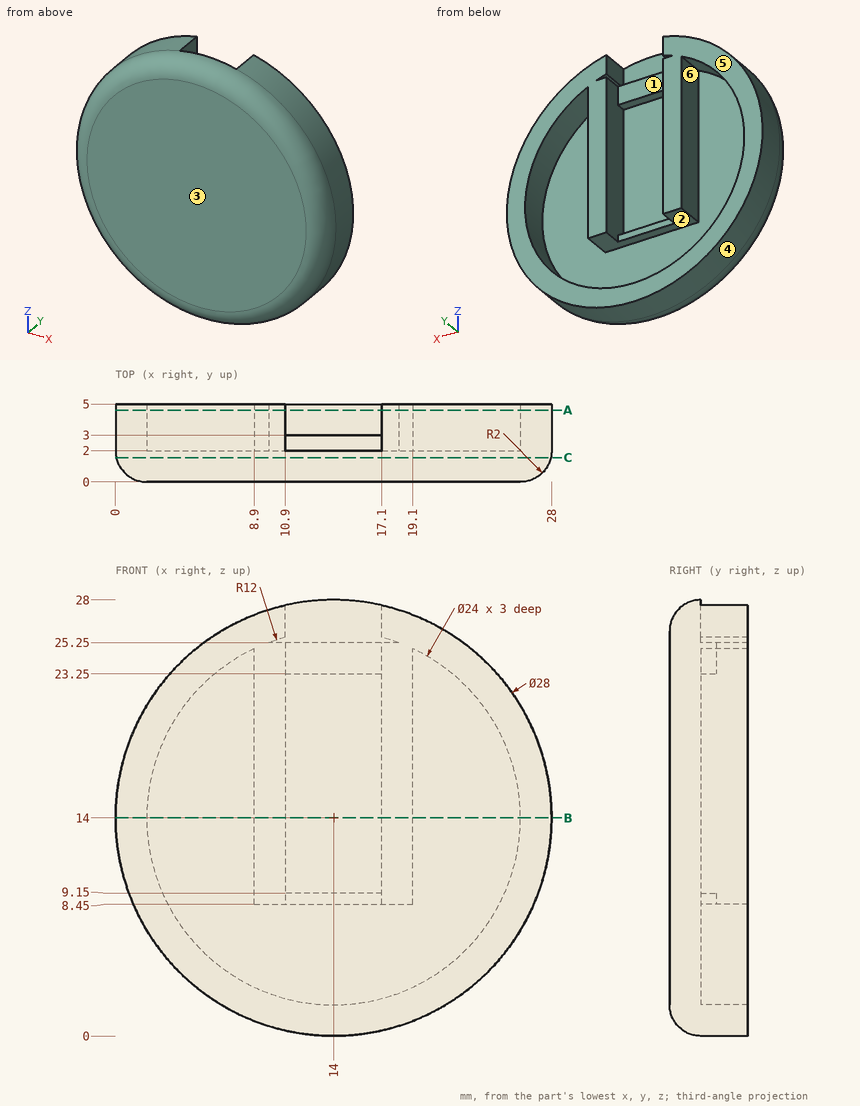
Answer from the drawing. Dimensions are ordinates in mm from the lowest x, y and z of the part. A direction names the side the tool comes from. Give positions to 0.01 mm unless a question says otherwise; leave off trailing zeros. Write each loop counter-clockwise with the first axis right and the second up, starting at its lowest first coordinate (ties: lowest second). Pieces come first, ordered by that corner, then holes.
1) Given P1, Ø0.8, axis at x = 15.5, z = 27, coming from the +Y side; P2, Ø0.6, axis at y = 3.5, z = 27, coming from the -X side; P3, Ø2, axis at x = 13.5, z = 24.5, coming from the +Y side, each flat-ended and moving along its own axis, determine where each tip first touches the part or whether it passes through.
2) Find the intervals of material crossed by L1, parallel to X at y = 4.25, z = 14; L2, parallel to Z at x = 14, y = 2.7; L3, parallel to X at y = 3.55, z = 17.75, in increasing order.
3) Section C-C (y = 1.55) is taken. Write down the section's boundary in (x, z).
4) For a pull along X with two mould halves and no side action, classify the marked faces 4, 5 and 6 as pulls with the +X half, pulls with the -X half, needs draft (parallel to the pull), parting line crosses it, or undercut.
5) Section B-B (z = 14) is taken. Write down the section's boundary in (x, y).
6) A tool of negligible diameter and unlimited length cuts with its end or side. For the marked faces 1, 2 and 3, from which of +Z, -Z, +X, -X, +Y, -Y can it reach the whole face along a straight path? Write none if from no direction.
7) Section A-A (y = 4.6) is taken. Write down the section's boundary in (x, z), and give its area (3 significant figures).
Response:
1. P1: stops at y = 2
1. P2: stops at x = 8.11
1. P3: stops at y = 3
2. L1: x = 0 to 2, 8.9 to 10.9, 17.1 to 19.1, 26 to 28
2. L2: z = 0 to 2, 8.45 to 9.15, 23.25 to 25.25
2. L3: x = 0.51 to 2.6, 8.9 to 10.9, 17.1 to 19.1, 25.4 to 27.49
3. outline: circle Ø27.9 at (14, 14)
4. face 4: parting line crosses it
4. face 5: needs draft
4. face 6: undercut
5. outline: (0, 2) arc R2 ccw to (2, 0) - (26, 0) arc R2 ccw to (28, 2) - (28, 5) - (26, 5) - (26, 2) - (19.1, 2) - (19.1, 5) - (17.1, 5) - (17.1, 2) - (10.9, 2) - (10.9, 5) - (8.9, 5) - (8.9, 2) - (2, 2) - (2, 5) - (0, 5) - close
6. face 1: +Z, +Y
6. face 2: +Y
6. face 3: +Z, -Z, +X, -X, -Y
7. outline: (8.9, 8.45) - (10.9, 8.45) - (10.9, 25.25) - (9.82, 25.25) arc R12 cw to (10.9, 25.59) - (10.9, 27.65) arc R14 ccw (long way) to (17.1, 27.65) - (17.1, 25.59) arc R12 cw to (18.18, 25.25) - (17.1, 25.25) - (17.1, 8.45) - (19.1, 8.45) - (19.1, 24.86) arc R12 cw (long way) to (8.9, 24.86) - close
7. area: 218 mm2
